Autodesk Fusion 360 part; units mm, degrees
sketch "Esquisse1" plane through (0, 0, 0) normal (0, 0, 1) x (1, 0, 0)
  line L0 (2, 0) -> (3.5, 0)
  line L1 (3.5, 0) -> (3.5, 15)
  line L2 (3.5, 15) -> (2, 15)
  line L3 (3.5, 0) -> (5.5, 0)
  line L4 (5.5, 0) -> (5.5, 15)
  line L5 (5.5, 15) -> (3.5, 15)
  line L6 (3.5, 15) -> (3.5, 0)
  line L7 (3.5, 15) -> (2.5, 15)
  line L8 (3.5, 15) -> (3.5, 14)
  line L9 (2.5, 15) -> (3.5, 14)
  line L10 (2.5, 13) -> (3.5, 14)
  line L11 (2.5, 13) -> (3.5, 12)
  line L12 (2.5, 11) -> (3.5, 12)
  line L13 (2.5, 7) -> (3.5, 8)
  line L14 (2.5, 9) -> (3.5, 8)
  line L15 (2.5, 9) -> (3.5, 10)
  line L16 (2.5, 11) -> (3.5, 10)
  line L17 (2.5, 1) -> (3.5, 0)
  line L18 (2.5, 1) -> (3.5, 2)
  line L19 (2.5, 3) -> (3.5, 2)
  line L20 (2.5, 3) -> (3.5, 4)
  line L21 (2.5, 5) -> (3.5, 4)
  line L22 (2.5, 5) -> (3.5, 6)
  line L23 (2.5, 7) -> (3.5, 6)
  line L24 (1.5, 7) -> (0.5, 8)
  line L25 (0.5, 15) -> (1.5, 15)
  line L26 (1.5, 9) -> (0.5, 8)
  line L27 (1.5, 15) -> (0.5, 14)
  line L28 (1.5, 11) -> (0.5, 10)
  line L29 (0.5, 15) -> (0.5, 14)
  line L30 (1.5, 1) -> (0.5, 0)
  line L31 (1.5, 5) -> (0.5, 4)
  line L32 (1.5, 3) -> (0.5, 2)
  line L33 (1.5, 7) -> (0.5, 6)
  line L34 (1.5, 13) -> (0.5, 12)
  line L35 (0.5, 0) -> (-1.5, 0)
  line L36 (1.5, 1) -> (0.5, 2)
  line L37 (1.5, 11) -> (0.5, 12)
  line L38 (1.5, 3) -> (0.5, 4)
  line L39 (1.5, 13) -> (0.5, 14)
  line L40 (1.5, 9) -> (0.5, 10)
  line L41 (1.5, 5) -> (0.5, 6)
  line L42 (0.5, 0) -> (0.5, 15)
  line L43 (-1.5, 15) -> (0.5, 15)
  line L44 (0.5, 15) -> (0.5, 0)
  line L45 (-1.5, 0) -> (-1.5, 15)
  line L46 (0.5, 15) -> (2, 15)
  line L47 (2, 0) -> (0.5, 0)
  dimension "d1" = 3.5
  dimension "d2" = 15
  dimension "d3" = 2
  dimension "d5" = 1
  dimension "d6" = 1
extrude "Extrusion1" add sketch "Esquisse1" against normal blind 2
extrude "Extrusion2" add sketch "Esquisse1" along normal blind 8 contours L1 L6 L17 L18 | L1 L3 L4 L5 L6 L8 | L30 L36 L42 L44 | L29 L35 L42 L43 L44 L45 | L1 L6 L19 L20 | L32 L38 L42 L44 | L1 L6 L21 L22 | L31 L41 L42 L44 | L1 L6 L13 L23 | L1 L2 L6 L7 L8 L9 | L25 L27 L29 L42 L44 L46 | L24 L33 L42 L44 | L1 L6 L14 L15 | L1 L6 L10 L11 | L34 L39 L42 L44 | L26 L40 L42 L44 | L1 L6 L12 L16 | L28 L37 L42 L44
fillet "Congé1" radius 0.5 10 edges at (5.5, 15, 3) (5.5, 7.5, -2) (2, 15, -2) (5.5, 0, 3) (2, 0, -2) (5.5, 7.5, 8) (4, 15, 8) (0, 15, 8) (4.5, 0, 8) (-0.5, 0, 8)
equation "d1 = ( 1.75 * 2 ) * 1 mm"
Geometry check sheet. Reference: the model listing, model coordinates, mm. A direction names the side the tool comes from. Round coordinates to 2 decimals unless told otherwise and drop trailing zeros. Order: outer loops, then holes, each group sorted by start corner. A loop starts at its lowest first (then second) coordinate and runs counter-clockwise, first axis right, second up. Notation, with made-up numbers: M 35,73 L 47,73 A18 ccw 47,86 Z; hole C -28,26.5 d1. An arc over 180 degrees is marked long. Answer in a Markdown table with one row per item. Add a question column.
Item 1: Draft check along Y on faces 3 (the face through (5.5, 7, 3)), 4 (the face through (0, 0, 3)), 5 (the face through (1, 9.5, 3.9)). Enter one of: released by +Y, released by -Y, zero draft, split by the parting line, or undercut.
Item 2: Set-up check for faces 1 (the face through (2, 8, -2)), 2 (the face through (3, 4.5, 3.9)): record each of +Z, -Z, +X, -X, +Y, -Y from which the full face is reachable in a straight line by a thin tool's end or side.
Item 3: Sectioned sample at B-B, the plane y = 11.5. Enter the section's corners in (x, z).
Item 4: Material ranges on L1, parallel to Z at x = 1.5, y = 9.25; L2, parallel to X at y = 8.5, z = 2.5; L3, parallel to X at y = 6.25, z = 1.5, recorded low to high. Write a range as [from, to].
Item 5: Sectioned sample at A-A, the plane y = 4.25. Enter the section's corners in (x, z).
Item 6: Depth check by flat-ended pin: pin 1 Ø2.5 at (x, y) = (2.5, 7.5) entering from +Z; pin 2 Ø2 at (x, y) = (2, 8) entering from +Z. Enter the tip coordinate at first touch or a pass-through.
Filled in:
| question | item | result |
|---|---|---|
| 1 | face 3 | zero draft |
| 1 | face 4 | released by -Y |
| 1 | face 5 | undercut |
| 2 | face 1 | -Z, +X, -X, +Y, -Y |
| 2 | face 2 | +Z |
| 3 | outline | M -1.5,-2 L 5,-2 A0.5 ccw 5.5,-1.5 L 5.5,7.5 A0.5 ccw 5,8 L 3,8 L 3,0 L 1,0 L 1,8 L -1.5,8 Z |
| 4 | L1 | z = [-2, 0] |
| 4 | L2 | x = [-1.5, 1], [3, 5.5] |
| 4 | L3 | x = [-1.5, 0.75], [3.25, 5.5] |
| 5 | outline | M -1.5,-2 L 5,-2 A0.5 ccw 5.5,-1.5 L 5.5,7.5 A0.5 ccw 5,8 L 3.25,8 L 3.25,0 L 0.75,0 L 0.75,8 L -1.5,8 Z |
| 6 | pin 1 | stops at z = 8 |
| 6 | pin 2 | stops at z = 0 |
